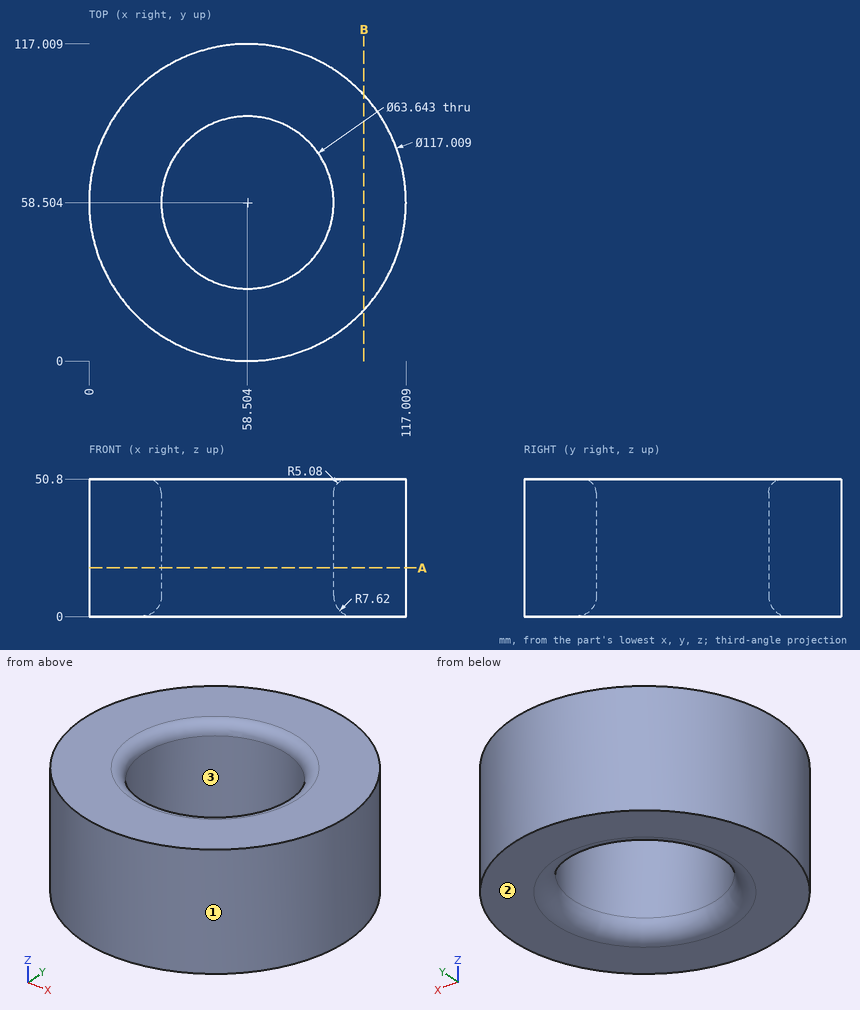
Can you work these out from the drawing? Everything is in mm from the part's minimum corner. Coordinates: 2 decimals unless noted, no trailing zeros. Loops run counter-clockwise (first coordinate to the right, second up) from the corner with the lowest first, then second, coordinate; pieces in that order, holes last. Notation, with made-up numbers: (84, 0.25) - (110, 0.25) arc R12 cw to (110, 10.25) - close; hole circle Ø5 at (60, 32.25). An arc over 180 degrees is marked (long way). Use a Markdown table: item, result.
Item 1: If I drill on probe 1 along Y at (x, z) = (62, 10) (1 decimal); probe 2 along X at (y, z) = (57, 16); probe 3 along Y at (x, z) = (65.5, 31), over which ranges is the centre line in solid material (lowest first)? Write a range as from..to.
Numbers:
| item | result |
|---|---|
| probe 1 | y = 0.1..26.9, 90.1..116.9 |
| probe 2 | x = 0.02..26.72, 90.29..116.99 |
| probe 3 | y = 0.42..27.46, 89.55..116.59 |
Item 2: We'd pull the mould along Y, two halves only. Please class the marked faces 1, 2 and 3: released by +Y, released by -Y, zero draft, split by the parting line, or undercut.
Numbers:
| item | result |
|---|---|
| face 1 | split by the parting line |
| face 2 | zero draft |
| face 3 | undercut |
Item 3: I want a section at A-A on z = 18. Please give me the cut outline in (x, y) (1 decimal).
Numbers:
| item | result |
|---|---|
| outline | circle Ø117 at (58.5, 58.5); hole circle Ø63.6 at (58.5, 58.5) |
Item 4: Will these pins go through, and if not, where does the flat tip stop? pin 1 (5 mm diameter, centred on x = 35.5, z = 36, fed in from -Y); pin 2 (1.5 mm diameter, centred on x = 73, z = 9.5, fed in from -Y); pin 3 (8 mm diameter, centred on x = 91, z = 29.5, fed in from +Y).
Numbers:
| item | result |
|---|---|
| pin 1 | stops at y = 3.71 |
| pin 2 | stops at y = 1.64 |
| pin 3 | stops at y = 109.6 |
Item 5: I want a section at B-B on x = 101.5. Please give me the cut outline in (y, z).
Numbers:
| item | result |
|---|---|
| outline | (18.83, 0) - (98.18, 0) - (98.18, 50.8) - (18.83, 50.8) - close |
